Could you check a few things on this drawing? It's one solid part, dimensions in mm from its lowest x, y, z. Give positions to 0.01 mm unless a question says otherwise; leave off trailing zeros. Order: outer loops, then holes, each group sorted by start corner. A loop starts at its lowest first (then second) coordinate and runs counter-clockwise, first axis right, second up. Notation, with made-up numbers: (34.5, 64.5) - (89.5, 64.5) arc R19 ccw to (89.5, 73.5) - close; hole circle Ø1 at (-34, 83.25). An arc over 180 degrees is marked (long way). Answer as CSV lines item,"result".
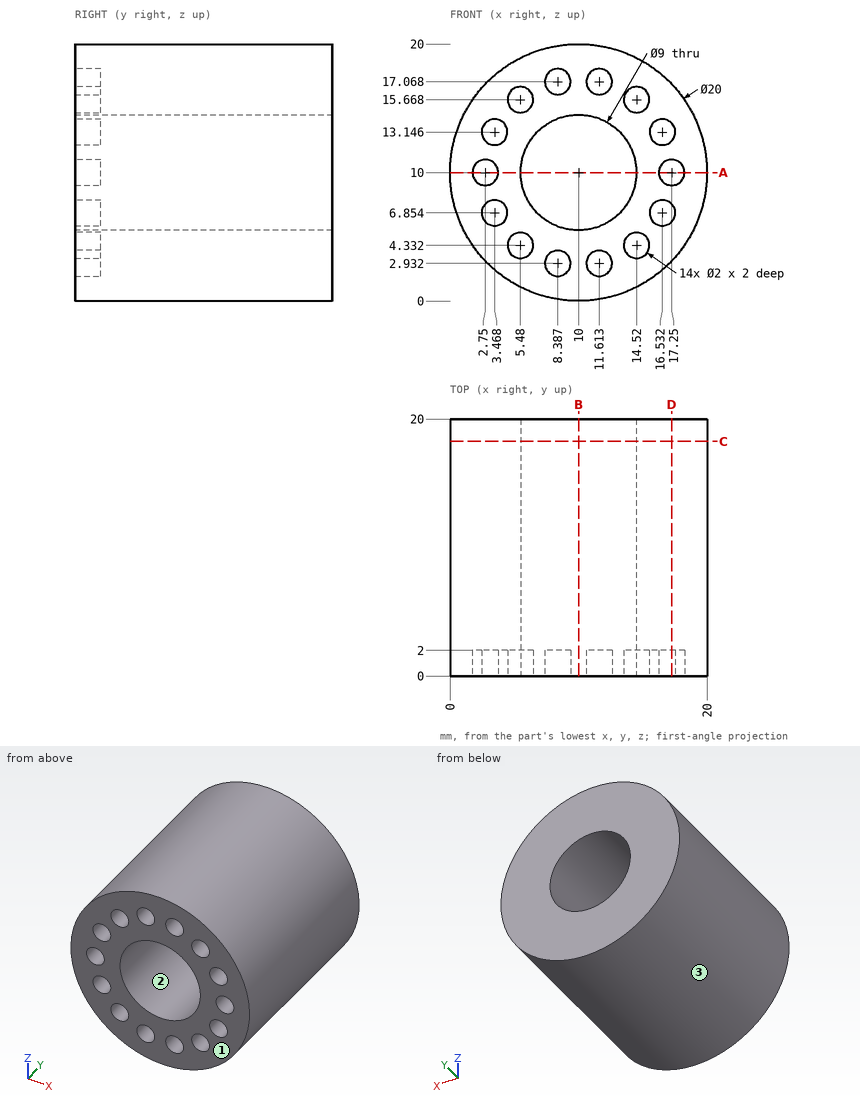
1) I need wall thicknesses on line 1 along X through (y, z) = (6.5, 10); line 2 along Z through (x, y) = (12, 11); line 3 along X through (y, z) = (2.75, 8.5). Which ranges of each line are inside material? Lowest first, please. Write a range as [from, to].
Answer block:
line 1,"[0, 5.5], [14.5, 20]"
line 2,"[0.2, 5.97], [14.03, 19.8]"
line 3,"[0.11, 5.76], [14.24, 19.89]"
2) I want a section at A-A on z = 10. Write out the boundary of the cut face in (x, y), plus the area to 3 significant figures.
Answer block:
outline,"(0, 0) - (1.75, 0) - (1.75, 2) - (3.75, 2) - (3.75, 0) - (5.5, 0) - (5.5, 20) - (0, 20) - close; (14.5, 0) - (16.25, 0) - (16.25, 2) - (18.25, 2) - (18.25, 0) - (20, 0) - (20, 20) - (14.5, 20) - close"
area,"212 mm2"
3) I'm going to push flat-ended pins straight in: P1, Ø12, axis at y = 16, z = 3, coming from the +X side; P2, Ø1, axis at x = 12, z = 17, coming from the -Y side; P3, Ø4, axis at x = 6.5, y = 8.5, coming from the -Z side. Where does each tip first touch, or does it pass through?
Answer block:
P1,"x = 19.95"
P2,"y = 2"
P3,"z = 0.11"
4) I want a section at D-D on x = 17.25. Write out the boundary of the cut face in (y, z).
Answer block:
outline,"(0, 3.11) - (20, 3.11) - (20, 16.89) - (0, 16.89) - (0, 13.84) - (2, 13.84) - (2, 12.45) - (0, 12.45) - (0, 11) - (2, 11) - (2, 9) - (0, 9) - (0, 7.55) - (2, 7.55) - (2, 6.16) - (0, 6.16) - close"
5) I want a section at B-B on x = 10. Write out the boundary of the cut face in (y, z).
Answer block:
outline,"(0, 0) - (20, 0) - (20, 5.5) - (0, 5.5) - close; (0, 14.5) - (20, 14.5) - (20, 20) - (0, 20) - close"
6) If we mould it in two halves opening along Z, with no side actions, what happens to the marked faces 1, 2 and 3? For each: +Z half, -Z half, draft (parallel to the pull), parting line (faces both ways), or undercut.
Answer block:
face 1,"draft"
face 2,"undercut"
face 3,"parting line"
7) I want a section at C-C on y = 18.25. Write out the boundary of the cut face in (x, z).
Answer block:
outline,"circle Ø20 at (10, 10); hole circle Ø9 at (10, 10)"
